Check sheet for the modelled part. Datum: model origin and axes. Units: mm. A direction names the side the tool comes from. Give positions to 0.01 mm unless a question says otherwise; leave off trailing zeros. Order: outer loops, then holes, each group sorted by start corner. A loop starts at its lowest first (then second) coordinate and runs counter-clockwise, first axis right, second up.
Autodesk Inventor part; units mm, degrees
ref_plane "YZ Plane" through (0, 0, 0) normal (1, 0, 0) x (0, 1, 0)
ref_plane "XZ Plane" through (0, 0, 0) normal (0, 1, 0) x (-1, 0, 0)
ref_plane "XY Plane" through (0, 0, 0) normal (0, 0, 1) x (1, 0, 0)
sketch "Sketch1" plane through (0, 0, 0) normal (0, 0, 1) x (1, 0, 0)
  line L0 (0, 0) -> (30, 0)
  line L1 (30, 0) -> (30, 50)
  line L2 (30, 50) -> (0, 50)
  line L3 (0, 50) -> (0, 0)
  dimension "d0" = 30
  dimension "d1" = 50
extrude "Extrusion1" add sketch "Sketch1" along normal blind 10
sketch "Sketch2" plane through (0, 0, 0) normal (0, -1, 0) x (1, 0, 0)
  line L0 (30, 0) -> (30, 10)
  line L1 (30, 0) -> (30, 1.5)
  line L2 (15, 0) -> (15, 12.0836) construction
  line L3 (30, 10) -> (30, 9) construction
  line L4 (30, 9) -> (-1.4785, 9) construction
  line L5 (27.4716, 5) -> (-0.9945, 5) construction
  line L6 (30, 5) -> (30.3, 5) construction
  line L7 (28.0716, 4.4) -> (30, 2.4716)
  line L8 (28.0716, 5.6) -> (30, 7.5284)
  line L9 (30, 5) -> (30, 5.6) construction
  line L10 (28.0716, 5.6) -> (25, 5.6)
  line L11 (25, 5.6) -> (25, 4.4)
  line L12 (25, 4.4) -> (28.0716, 4.4)
  arc A0 (30, 6.9774) -> (28.8858, 6.4142) centre (30.3, 5) ccw construction
  arc A1 (28.3921, 4.4) -> (28.8858, 3.5858) centre (30.3, 5) ccw construction
  line L13 (1.9284, 4.4) -> (0, 2.4716)
  line L14 (1.9284, 5.6) -> (0, 7.5284)
  line L15 (1.9284, 5.6) -> (5, 5.6)
  line L16 (5, 5.6) -> (5, 4.4)
  line L17 (5, 4.4) -> (1.9284, 4.4)
  line L18 (30, 10) -> (0, 10)
  line L19 (0, 0) -> (0, 10)
  line L20 (0, 10) -> (0, 0)
  line L21 (30, 0) -> (30, -3)
  line L22 (30, -3) -> (0, -3)
  line L23 (0, -3) -> (0, 0)
  line L24 (30, 0) -> (0, 0)
  line L25 (0, 0) -> (30, 0)
  circle A2 centre (15, 5) radius 1.5
  line L26 (4, 4.4) -> (4, 5.6)
  line L27 (25, 4.4) -> (26, 4.4)
  line L28 (26, 4.4) -> (26, 5.6)
  line L29 (25, 5.6) -> (25, 4.4)
  point P0 (4, 5)
  dimension "d4" = 1.5
  dimension "d7" = 1
  dimension "d9" = 0.3
  dimension "d11" = 90
  dimension "d12" = 0.6
  dimension "d13" = 5
  dimension "d14" = 1.2
  dimension "d27" = 3
  dimension "d31" = 3
  dimension "d90" = 5
  dimension "d91" = 4
  dimension "d94" = 1
extrude "Extrusion3" cut sketch "Sketch2" against normal blind 50 contours L7 L12 L28 L10 L8 L0 | L19 L14 L15 L26 L17 L13
sketch "Sketch4" plane through (0, 0, 0) normal (0, -1, 0) x (1, 0, 0)
  line L0 (30, 0) -> (0, 0)
  line L1 (30, 0) -> (0, 0)
  line L2 (0, 0) -> (0, -6)
  line L3 (0, -6) -> (30, -6)
  line L4 (30, -6) -> (30, 0)
  dimension "d28" = 6
extrude "Extrusion5" add sketch "Sketch4" against normal blind 50
sketch "Sketch5" plane through (1.9284, 0, 5.6) normal (0, -1, 0) x (1, 0, 0)
  line L0 (23.0716, -1.2) -> (23.0716, 0)
  line L1 (23.0716, -0.6) -> (3.0716, -0.6) construction
  line L2 (19.0716, 2.4) -> (7.0716, 2.4)
  line L3 (13.0716, 2.4) -> (13.0716, -11.6) construction
  line L4 (-1.9284, -11.6) -> (28.0716, -11.6)
  line L5 (13.0716, 2.4) -> (13.0716, -4.1)
  line L6 (13.0716, -4.1) -> (-1.9284, -4.1) construction
  line L7 (-1.9284, -11.6) -> (-1.9284, -3.1284) construction
  point P0 (-1.9284, -5.6)
  dimension "d33" = 6.5
ref_plane "Work Plane1" through (30, 0, -6) normal (0, 0, -1) x (-1, 0, 0)
sketch "Sketch7" plane through (25, 50, 5.6) normal (0, 1, 0) x (1, 0, 0)
  line L0 (-25, -1.9284) -> (-23.0716, 0)
  line L1 (-25, 11.6) -> (-25, 3.1284)
  line L2 (-25, -1.9284) -> (-25, 3.1284)
  line L3 (-23.0716, 1.2) -> (-25, 3.1284)
  line L4 (-25, 3.1284) -> (-23.0716, 1.2)
  line L5 (-20, 0) -> (-20, 1.2)
  line L6 (-23.0716, 1.2) -> (-20, 1.2)
  line L7 (-20, 1.2) -> (-20, 0)
  line L8 (-20, 0) -> (-23.0716, 0)
  line L9 (-23.0716, 0) -> (-25, -1.9284)
  line L10 (0, 0) -> (0, 1.2)
  line L11 (0, 0) -> (0, 1.2)
  line L12 (0, 1.2) -> (3.4081, 1.2)
  line L13 (3.0716, 1.2) -> (5, 3.1284)
  line L14 (5, 3.1284) -> (3.0716, 1.2)
  line L15 (3.0716, 0) -> (1, 0)
  line L16 (0, 0) -> (3.0716, 0)
  line L17 (5, -1.9284) -> (3.0716, 0)
  line L18 (3.0716, 0) -> (5, -1.9284)
  line L19 (5, -1.9284) -> (5, 3.1284)
  point P0 (-25, 5.6)
sketch "Sketch8" plane through (1.9284, 0, 5.6) normal (0, -1, 0) x (1, 0, 0)
  line L0 (28.0716, 1.9284) -> (28.0716, 4.4)
  line L1 (28.0716, 1.9284) -> (28.0716, -3.1284)
  line L2 (28.0716, -3.1284) -> (26.1431, -1.2)
  line L3 (23.0716, -1.2) -> (23.0716, 0)
  line L4 (26.1431, -1.2) -> (23.0716, -1.2)
  line L5 (23.0716, -1.2) -> (23.0716, 0)
  line L6 (23.0716, 0) -> (26.1431, 0)
  line L7 (26.1431, 0) -> (28.0716, 1.9284)
  line L8 (13.0716, -3.7758) -> (13.0716, 8.1492) construction
  line L9 (-1.9284, -3.1284) -> (0, -1.2)
  line L10 (-1.9284, 1.9284) -> (-1.9284, -3.1284)
  line L11 (3.0716, -1.2) -> (3.0716, 0)
  line L12 (0, -1.2) -> (3.0716, -1.2)
  line L13 (3.0716, 0) -> (0, 0)
  line L14 (0, 0) -> (-1.9284, 1.9284)
  line L15 (23.0716, -1.2) -> (24.0716, -1.2)
  line L16 (24.0716, -1.2) -> (24.0716, 0)
  line L17 (23.0716, 0) -> (23.0716, -1.2)
  point P0 (-1.9284, -5.6)
  dimension "d93" = 1
sketch "Sketch10" plane through (30, 0, -6) normal (0, 0, -1) x (-1, 0, 0)
  line L0 (0, 50) -> (30, 50) construction
  line L1 (0, 50) -> (7.5, 50) construction
  line L2 (7.5, 50) -> (7.5, 32.5) construction
  line L3 (30, 50) -> (22.5, 50) construction
  line L4 (22.5, 50) -> (22.5, 32.5) construction
  line L5 (30, 0) -> (0, 0) construction
  line L6 (0, 0) -> (7.5, 0) construction
  line L7 (7.5, 0) -> (7.5, 17.5) construction
  line L8 (30, 0) -> (22.5, 0) construction
  line L9 (22.5, 0) -> (22.5, 17.5) construction
  line L10 (21, 50) -> (9, 50) construction
  line L11 (15, 50) -> (15, 25) construction
  line L12 (0, 0) -> (0, 50) construction
  line L13 (15, 25) -> (0, 25)
  point P0 (0, 5)
  point P1 (0, 45)
  dimension "d53" = 7.5
  dimension "d54" = 17.5
  dimension "d55" = 7.5
  dimension "d56" = 17.5
  dimension "d57" = 7.5
  dimension "d58" = 17.5
  dimension "d59" = 7.5
  dimension "d60" = 17.5
hole "Hole2" at (22.5, 17.5, -6) at (7.5, 17.5, -6) at (7.5, 32.5, -6) at (22.5, 32.5, -6) at (15, 25, -6) direction (0, 0, 1) diameter 1.567 end through all
sketch "Sketch11" plane through (30, 0, -6) normal (0, 0, -1) x (-1, 0, 0)
  circle A0 centre (22.5, 32.5) radius 0.7835
  circle A1 centre (7.5, 32.5) radius 0.7835
  point P0 (30, 0)
  point P1 (22.5, 12.5)
  point P2 (7.5, 12.5)
  point P3 (22.5, 27.5)
  point P4 (7.5, 27.5)
  dimension "d68" = 20
  dimension "d76" = 15
hole "Hole3" at (7.5, 12.5, -6) at (22.5, 12.5, -6) at (7.5, 27.5, -6) at (22.5, 27.5, -6) direction (0, 0, 1) diameter 4.2 end through all
chamfer "Chamfer1" distance 0.3 angle 45 5 edges at (7.5, 31.7165, -6) (7.5, 16.7165, -6) (22.5, 16.7165, -6) (22.5, 31.7165, -6) (15, 24.2165, -6)
sketch "Sketch12" plane through (0, 0, 10) normal (0, -1, 0) x (1, 0, 0)
  line L0 (30, -2.4716) -> (30, 0)
  line L1 (30, 0) -> (30, -2)
  line L2 (30, -2) -> (0, -2)
  line L3 (30, -2) -> (30, 0)
  line L4 (0, 0) -> (30, 0)
  line L5 (0, 0) -> (0, -2)
  line L6 (0, -2.4716) -> (0, 0)
  point P0 (0, -10)
  dimension "d80" = 2
extrude "Extrusion10" cut sketch "Sketch12" against normal through all
chamfer "Chamfer2" distance 0.3 angle 45 1 edges at (15, 24.2165, -5.7)
sketch "Sketch13" plane through (25, 50, 5.6) normal (0, 1, 0) x (1, 0, 0)
  line L0 (-8.9165, 11.6) -> (-11.0835, 11.6) construction
  line L1 (-10, 11.6) -> (-10, 3.4303) construction
  point P0 (-25, 5.6)
sketch "Sketch14" plane through (25, 50, 5.6) normal (0, 1, 0) x (1, 0, 0)
  line L0 (-10.7835, -2.4) -> (-9.2165, -2.4)
  line L1 (-10, -2.4) -> (-10, 4.1)
  circle A0 centre (-10, 4.1) radius 5
  point P0 (-25, 5.6)
  dimension "d86" = 6.5
  dimension "d87" = 10
extrude "Extrusion11" cut sketch "Sketch14" against normal blind 17
sketch "Sketch15" plane through (25, 0, 4.4) normal (0, -1, 0) x (1, 0, 0)
  line L0 (3.0716, 0) -> (1, 0)
  line L1 (0, 0) -> (1, 0)
  line L2 (1, 0) -> (1, 1.2)
  line L3 (1, 1.2) -> (3.0716, 1.2)
  line L4 (1, 0) -> (0, 0)
  line L5 (0, 0) -> (0, 1.2)
  line L6 (0, 1.2) -> (1, 1.2)
  point P0 (-25, -4.4)
  dimension "d92" = 1
equation "\"d54\" = d56"
equation "\"d58\" = d56"
equation "\"d60\" = d56"
properties part number "Platform" material "Steel, Carbon"
(1) Sectioned sample at A-A (y = 32.5). Enter the section's corners in (x, z).
(2) Go/stop test with flat-tipped pins: P1, Ø4, axis at x = 7.5, y = 12.5, coming from the -Z side; P2, Ø3, axis at x = 15.5, z = 1, coming from the +Y side; P3, Ø0.6, axis at y = 25.5, z = 5, coming from the -X side. Record where each tip stops, or that it passes through.
(3) Sectioned sample at B-B (z = 1.5). Count the separate pieces of the cut face and the enclosed holes in it, plus the area to 3 significant figures.
(4) Release check for a two-part mould opening along Z. For faces 1 (the face through (6.081, 25.952, 1.098)), 2 (the face through (0.98, 24.65, 6.55)), 3 (the face through (19, 25, 8)) record: released by +Z, released by -Z, zero draft, split by the parting line, or undercut.
(5) Tool access check on faces 4 (the face through (27, 25, 5.6)), 5 (the face through (8.265, 17.33, 1.246)), 6 (the face through (3, 25, 4.4)). Record the directions out of +Z, -Z, +X, -X, +Y, -Y that give a thin tool (end or side, any length) a straight path to the whole face; none if there is none.
(6) Thickness scan on L1, parallel to X at y = 17.5, z = -4; L2, parallel to Y at x = 22.5, z = 5.25; L3, parallel to X at y = 12, z = 5.5. Record the ranges inside material, lowest first.
(7) Sectioned sample at C-C (y = 38.5). Enter the section's corners in (x, z), plus the area to 3 significant figures.
(8) Sectioned sample at D-D (x = 7.5). Enter the section's corners in (y, z).
Values follow:
1. outline: (0, -6) - (6.42, -6) - (6.72, -5.7) - (6.72, 8) - (0, 8) - (0, 7.53) - (1.93, 5.6) - (4, 5.6) - (4, 4.4) - (1.93, 4.4) - (0, 2.47) - close; (8.28, -5.7) - (8.58, -6) - (21.42, -6) - (21.72, -5.7) - (21.72, 8) - (8.28, 8) - close; (23.28, -5.7) - (23.58, -6) - (30, -6) - (30, 2.47) - (28.07, 4.4) - (26, 4.4) - (26, 5.6) - (28.07, 5.6) - (30, 7.53) - (30, 8) - (23.28, 8) - close
2. P1: passes through
2. P2: stops at y = 33
2. P3: stops at x = 4
3. separate pieces: 1
3. enclosed holes: 9
3. area: 1,260 mm2
4. face 1: zero draft
4. face 2: undercut
4. face 3: released by +Z
5. face 4: +X, +Y, -Y
5. face 5: +Z, -Z
5. face 6: -X, +Y, -Y
6. L1: x = 0 to 6.72, 8.28 to 21.72, 23.28 to 30
6. L2: y = 0 to 10.4, 14.6 to 16.72, 18.28 to 25.4, 29.6 to 31.72, 33.28 to 50
6. L3: x = 4 to 5.46, 9.54 to 20.46, 24.54 to 26
7. outline: (0, -6) - (30, -6) - (30, 2.47) - (28.07, 4.4) - (26, 4.4) - (26, 5.6) - (28.07, 5.6) - (30, 7.53) - (30, 8) - (0, 8) - (0, 7.53) - (1.93, 5.6) - (4, 5.6) - (4, 4.4) - (1.93, 4.4) - (0, 2.47) - close; hole circle Ø10 at (15, 1.5)
7. area: 324 mm2
8. outline: (0, -6) - (10.4, -6) - (10.4, 8) - (0, 8) - close; (14.6, -6) - (16.42, -6) - (16.72, -5.7) - (16.72, 8) - (14.6, 8) - close; (18.28, -5.7) - (18.58, -6) - (25.4, -6) - (25.4, 8) - (18.28, 8) - close; (29.6, -6) - (31.42, -6) - (31.72, -5.7) - (31.72, 8) - (29.6, 8) - close; (33.28, -5.7) - (33.58, -6) - (50, -6) - (50, 8) - (33.28, 8) - close
